Autodesk Inventor part; units mm, degrees
ref_plane "YZ Plane" through (0, 0, 0) normal (1, 0, 0) x (0, 1, 0)
ref_plane "XZ Plane" through (0, 0, 0) normal (0, 1, 0) x (-1, 0, 0)
ref_plane "XY Plane" through (0, 0, 0) normal (0, 0, 1) x (1, 0, 0)
sketch "Sketch1" plane through (0, 0, 0) normal (0, 1, 0) x (-1, 0, 0)
  line L0 (-1.5, 7) -> (-1.5, -13)
  line L1 (-1.5, -13) -> (0, -13)
  line L2 (0, -13) -> (0, 0)
  line L3 (0, 0) -> (2.4, 0)
  line L4 (2.4, 0) -> (2.4, -10)
  line L5 (2.4, -10) -> (0.4, -10)
  line L6 (0.4, -10) -> (0.4, -13)
  line L7 (0.4, -13) -> (10.4, -13)
  line L8 (10.4, -13) -> (10.4, 62)
  line L9 (10.4, 62) -> (7.4, 62)
  line L10 (7.4, 62) -> (2.4, 7)
  line L11 (2.4, 7) -> (-1.5, 7)
  dimension "d0" = 0.4
  dimension "d1" = 2
  dimension "d2" = 10
  dimension "d3" = 75
  dimension "d4" = 7
  dimension "d5" = 10
  dimension "d6" = 3
  dimension "d7" = 1.5
  dimension "d14" = 3
extrude "Extrusion1" add sketch "Sketch1" along normal blind 10
mirror "Mirror1" about plane through (1.5, 0, 7) normal (1, 0, 0) of "Extrusion1"
chamfer "Chamfer1" distance 8 angle 45 5 edges at (-5.4, 10, -13) (1.5, 10, -13) (8.4, 10, -13) (13.4, 5, -13) (-10.4, 5, -13)
fillet "Fillet1" radius 1 12 edges at (-0.4, 1, -13) (0, 1, -13) (3.4, 1, -13) (3, 1, -13) (-0.4, 2.5, -10) (3.4, 2.5, -10) (5.4, 5, 0) (3, 5, 0) (0, 5, 0) (-2.4, 5, 0) (-2.4, 5, 7) (5.4, 5, 7)
properties part number "adjuster grip"
Part model, mm, in its own coordinate system. A direction names the side the tool comes from. Round coordinates to 2 decimals unless told otherwise and drop trailing zeros. Write each loop counter-clockwise with the first axis right and the second up, starting at its lowest first coordinate (ties: lowest second). Pieces come first, ordered by that corner, then holes. Notation, with made-up numbers: (34.25, 80.25) - (39.25, 80.25) arc R20 ccw to (39.25, 108.25) - close; hole circle Ø10 at (45.5, 64). An arc over 180 degrees is marked (long way). Use CSV: the item, a comma, the result in double quotes.
Item 1: Slice it at D-D, the plane z = 31. Write the cut outline in (x, y).
Results list:
outline,"(-10.4, 0) - (-4.58, 0) - (-4.58, 10) - (-10.4, 10) - close; (7.58, 0) - (13.4, 0) - (13.4, 10) - (7.58, 10) - close"
Item 2: Pull direction Z, two halves, no side cores. Call faces 6 (the flat face through (0, 4, -5)), 7 (the flat face through (-4, 7, -8)), 8 (the flat face through (-2.4, 5, -5)): pulls with the +Z half, pulls with the -Z half, needs draft (parallel to the pull), parting line crosses it, or undercut.
Results list:
face 6,"needs draft"
face 7,"pulls with the -Z half"
face 8,"undercut"
Item 3: Wall check: L1, parallel to X at y = 3.5, z = -8; L2, parallel to X at y = 0.5, z = -3; L3, parallel to X at y = 7, z = 44.5. Give the ranges that are in metal, low to high.
Results list:
L1,"x = -7.4 to -2.4, 0 to 3, 5.4 to 10.4"
L2,"x = -10.4 to -2.4, 0 to 3, 5.4 to 13.4"
L3,"x = -10.4 to -5.81, 8.81 to 13.4"
Item 4: Tool access for faces 1 (the flat face through (5.4, 5, -6)), 2 (the flat face through (7, 0, 17)), 3 (the flat face through (12, 5, 62)), 4 (the flat face through (-4.976, 4.93, 35.333)), 5 (the flat face through (3, 4, -5)): list every direction of +Z, -Z, +X, -X, +Y, -Y with a clear straight run to the whole face (end or side of a thin tool).
Results list:
face 1,"+Y, -Y"
face 2,"+Z, -Z, +X, -X, -Y"
face 3,"+Z, +X, -X, +Y, -Y"
face 4,"+Z, +Y, -Y"
face 5,"-Z, +Y, -Y"
Item 5: Flat gauge pins, fed straight in: P1, Ø0.5, axis at x = -2, y = 3.5, coming from the +Z side; P2, Ø0.8, axis at y = 1.5, z = -11.5, coming from the -X side; P3, Ø5, axis at x = 0, y = 3, coming from the -Z side; P4, Ø1.8, axis at x = 1.5, y = 2.5, coming from the +Z side. Where does each tip first touch, or does it go through?
Results list:
P1,"stops at z = 7.35"
P2,"stops at x = -4.3"
P3,"stops at z = -13"
P4,"stops at z = 7"
Item 6: Slice it at B-B, the plane y = 8. Write the cut outline in (x, z).
Results list:
outline,"(-10.4, -5) - (-8.4, -7) - (-2.4, -7) - (-2.4, -1) arc R1 cw to (-1.4, 0) - (-1, 0) arc R1 cw to (0, -1) - (0, -7) - (3, -7) - (3, -1) arc R1 cw to (4, 0) - (4.4, 0) arc R1 cw to (5.4, -1) - (5.4, -7) - (11.4, -7) - (13.4, -5) - (13.4, 62) - (10.4, 62) - (5.48, 7.91) arc R1 cw to (4.49, 7) - (-1.49, 7) arc R1 cw to (-2.48, 7.91) - (-7.4, 62) - (-10.4, 62) - close"
Item 7: Slice it at A-A, the plane z = 45. Write the cut outline in (x, y), then the cut area to 3 significant figures.
Results list:
outline,"(-10.4, 0) - (-5.85, 0) - (-5.85, 10) - (-10.4, 10) - close; (8.85, 0) - (13.4, 0) - (13.4, 10) - (8.85, 10) - close"
area,"90.9 mm²"
Item 8: Slice it at C-C, the plane x = -4. Write the cut outline in (y, z), then the cut area to 3 significant figures.
Results list:
outline,"(0, -11.4) - (3.6, -11.4) - (10, -5) - (10, 24.6) - (0, 24.6) - close"
area,"340 mm²"
